Read the model definition and answer for the solid it produces. Units are mm, in the model's axes. Give positions to 0.01 mm unless a question says otherwise; leave off trailing zeros. Order: outer loops, then holes, each group sorted by start corner. A loop starts at its lowest first (then second) coordinate and runs counter-clockwise, first axis right, second up. Notation, with made-up numbers: (-8.75, 24) - (7.25, 24) arc R21 cw to (7.25, 41) - close; hole circle Ø1 at (77, 68). An arc over 180 degrees is marked (long way). Write each question's results on one line, items separated by ' | '. Start each with the question number.
Q1. Find section A-A on x = 777. Give the vertices of the cut face in (y, z) (3 decimals), and give its area (3 significant figures).
Q2. Find the intervals of material crossed by line 1 along Y through (x, z) = (764.5, 1.75); line 2 along Y through (x, z) = (807, -8.25); line 3 along Z through (x, y) = (915, 21.25), in increasing order. Write a range as from..to.
Q3. Flat-ended cylindrical pins translate along their axes: P1, Ø11, axis at x = 406.5, y = 9, coming from the +Z side; P2, Ø1.5, axis at x = 1077.5, y = 20.5, coming from the +Z side; P3, Ø3, axis at x = 247.5, y = 12.5, coming from the -Z side. Find the tip coordinate at first contact, or state that the pin passes through.
Q4. Find section B-B on y = 12.25. Give the vertices of the cut face in (x, z).
from build123d import *

# Parameters (mm, degrees)
BOSS_EXTRUDE1_DEPTH = 1524


with BuildPart() as part:
    # Sketch1 → Boss-Extrude1 (new body)
    with BuildSketch(Plane(origin=(0, 0, 0), x_dir=(0, 0, -1), z_dir=(1, 0, 0))):
        with BuildLine():
            Line((9.525, 0), (-9.525, 0))
            Line((-9.525, 0), (-9.525, 0.508))
            Line((-9.525, 0.508), (-0.715679151, 2.141916092))
            ThreePointArc((-0.715679151, 2.141916092), (-0.566703436, 2.229252122), (-0.508, 2.391656716))
            Line((-0.508, 2.391656716), (-0.508, 16.142634631))
            ThreePointArc((-0.508, 16.142634631), (-0.963665934, 17.594237711), (-2.167174412, 18.525017111))
            Line((-2.167174412, 18.525017111), (-4.6863, 19.4564))
            Line((-4.6863, 19.4564), (-4.6863, 21.1074))
            ThreePointArc((-4.6863, 21.1074), (-4.239930735, 22.185030735), (-3.1623, 22.6314))
            Line((-3.1623, 22.6314), (3.1623, 22.6314))
            ThreePointArc((3.1623, 22.6314), (4.239930735, 22.185030735), (4.6863, 21.1074))
            Line((4.6863, 21.1074), (4.6863, 19.4564))
            Line((4.6863, 19.4564), (2.167174412, 18.525017111))
            ThreePointArc((2.167174412, 18.525017111), (0.963665934, 17.594237711), (0.508, 16.142634631))
            Line((0.508, 16.142634631), (0.508, 2.391656716))
            ThreePointArc((0.508, 2.391656716), (0.566703436, 2.229252122), (0.715679151, 2.141916092))
            Line((0.715679151, 2.141916092), (9.525, 0.508))
            Line((9.525, 0.508), (9.525, 0))
        make_face()
    extrude(amount=BOSS_EXTRUDE1_DEPTH)


solid = part.part
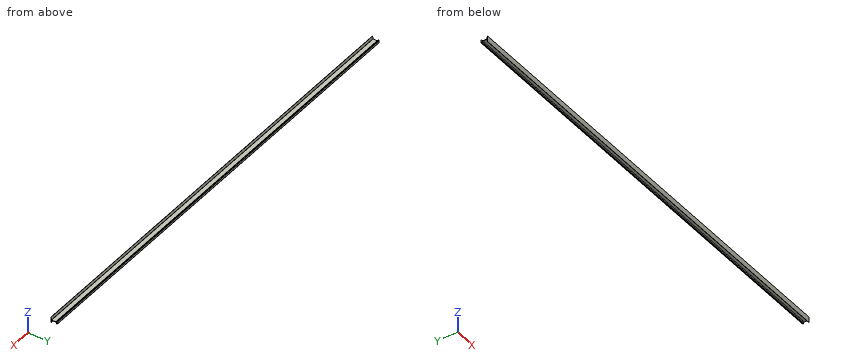
Working result:
1) outline: (0, -9.525) - (0.508, -9.525) - (2.142, -0.716) arc R0.254 cw to (2.392, -0.508) - (16.143, -0.508) arc R2.54 cw to (18.525, -2.167) - (19.456, -4.686) - (21.107, -4.686) arc R1.524 ccw to (22.631, -3.162) - (22.631, 3.162) arc R1.524 ccw to (21.107, 4.686) - (19.456, 4.686) - (18.525, 2.167) arc R2.54 cw to (16.143, 0.508) - (2.392, 0.508) arc R0.254 cw to (2.142, 0.716) - (0.508, 9.525) - (0, 9.525) - close | area: 80.4 mm²
2) line 1: 0..1.95, 18.33..22.63 | line 2: 0..0.74 | line 3: -4.68..4.68
3) P1: z = 0.51 | P2: z = 4.69 | P3: z = -0.51
4) outline: (0, -0.51) - (1524, -0.51) - (1524, 0.51) - (0, 0.51) - close
